Geometry: final body of the model. Coordinates: model frame, mm. Face numbers are marked on the shaded views. A direction names the side the tool comes from. Give positions to 0.01 mm unless a question says otherwise; leave off trailing zeros. Loops run counter-clockwise (first coordinate to the right, second up) from the corner with the lowest first, then second, coordinate; pieces in that order, holes last. Notation, with made-up numbers: (38, 37.25) -> (86, 37.25) arc R17 ccw to (86, 64.25) -> close; hole circle Ø4 at (-15.5, 10.25). An arc over 180 degrees is marked (long way). Answer in a Markdown table with one row per item. Add a question column.
1) Section query A-A (x = 42.5). Return the cut outline in (y, z).
2) Section query C-C (x = 29.5). Return the cut outline in (y, z).
3) Line query: line 1 (X direction, y = 75.75, z = 15); line 2 (Z direction, x = 42, y = 73); line 3 (Z direction, x = 21, y = 32). Output: solid intervals per line, ascending. Write a range as from..to.
4) Section query B-B (z = 15). Return the cut outline in (x, y).
5) First-contact query: P1, Ø3, axis at y = 74.5, z = 18.5, coming from the -X side; P2, Ø6.5, axis at x = 17.5, z = 15, coming from the +Y side; P3, Ø6, axis at x = -15.5, y = 21.5, coming from the -Z side; P4, Ø5.5, axis at x = 30, z = 14.5, coming from the -Y side. Flat tips, straight axial feed; report the tip coordinate or a pass-through.
6) Access query for the marked faces 1 and 2. Directions: +Z, -Z, +X, -X, +Y, -Y. A direction counts if a zero-diameter tool reaches every point of the face in a straight line with its end or side. Return the directions, or none.
7) Section query D-D (y = 2). Return the cut outline in (x, z).
```python
from build123d import *

# Parameters (mm, degrees)
SKETCH_1_W          = 100
SKETCH_1_H          = 160
EXTRUDE_1_DEPTH     = 5
SKETCH_2_W          = 40
SKETCH_2_H          = 20
EXTRUDE_2_DEPTH     = 10
SKETCH_3_R          = 4
CUT_EXTRUDE_1_DEPTH = 10
FILLET_1_R          = 2


with BuildPart() as part:
    # 草图1 → 凸台-拉伸1 (new body)
    with BuildSketch(Plane.XY):
        Rectangle(SKETCH_1_W, SKETCH_1_H)
    extrude(amount=EXTRUDE_1_DEPTH)

    # 草图2 → 凸台-拉伸2 (add)
    with BuildSketch(Plane(origin=(0, 80, 0), x_dir=(1, 0, 0), z_dir=(0, 1, 0))):
        with Locations((30, -15)):
            Rectangle(SKETCH_2_W, SKETCH_2_H)
    extrude(amount=-EXTRUDE_2_DEPTH)

    # 草图3 → 切除-拉伸1 (cut)
    with BuildSketch(Plane.XZ.offset(-70)):
        with Locations(Location((17.5, 15, 0), (0, 0, 270))):
            Circle(SKETCH_3_R)
        with Locations(Location((42.5, 15, 0), (0, 0, 270))):
            Circle(SKETCH_3_R)
    extrude(amount=-CUT_EXTRUDE_1_DEPTH, mode=Mode.SUBTRACT)

    # 圆角1
    fillet_1_edges = [part.edges().sort_by_distance(p)[0] for p in [
        (30, 70, 5),
        (10, 75, 5),
    ]]
    fillet(fillet_1_edges, radius=FILLET_1_R)


solid = part.part
```
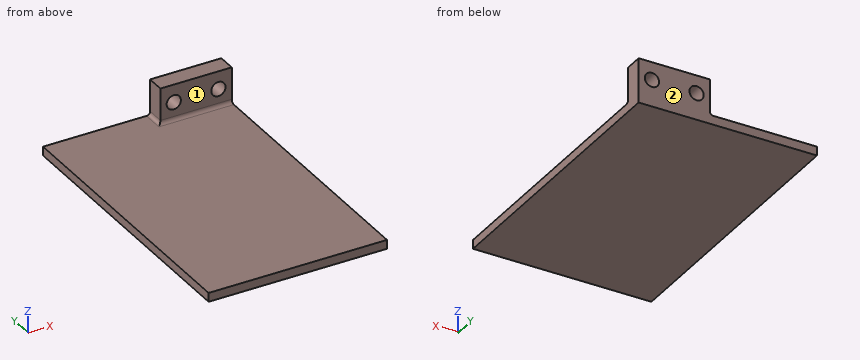
Evaluation:
| question | item | result |
|---|---|---|
| 1 | outline | (-80, 0) -> (80, 0) -> (80, 11) -> (70, 11) -> (70, 7) arc R2 cw to (68, 5) -> (-80, 5) -> close; (70, 19) -> (80, 19) -> (80, 25) -> (70, 25) -> close |
| 2 | outline | (-80, 0) -> (80, 0) -> (80, 25) -> (70, 25) -> (70, 7) arc R2 cw to (68, 5) -> (-80, 5) -> close |
| 3 | line 1 | 10..13.5, 21.5..38.5, 46.5..50 |
| 3 | line 2 | 0..11.03, 18.97..25 |
| 3 | line 3 | 0..5 |
| 4 | outline | (10, 70) -> (13.5, 70) -> (13.5, 80) -> (10, 80) -> close; (21.5, 70) -> (38.5, 70) -> (38.5, 80) -> (21.5, 80) -> close; (46.5, 70) -> (50, 70) -> (50, 80) -> (46.5, 80) -> close |
| 5 | P1 | x = 10 |
| 5 | P2 | through |
| 5 | P3 | z = 0 |
| 5 | P4 | y = 70 |
| 6 | face 1 | +Z, +X, -X, -Y |
| 6 | face 2 | +Z, -Z, +X, -X, +Y |
| 7 | outline | (-50, 0) -> (50, 0) -> (50, 5) -> (-50, 5) -> close |
